from build123d import *

# Parameters (mm, degrees)
F0_W        = 50.1185376197
F0_H        = 40.0948291644
F1_DEPTH    = 50
F2_T        = -2.5
F3_T1_DEPTH = 75
F4_T1_DEPTH = 75


# Not quite as in the source:
# - a fillet or chamfer that OpenCascade refuses, or shapes differently, is made with other operations: its cross-section is extruded or revolved along the edge and cut away or added


with BuildPart() as f1:
    # F0 (on Front) → F1 (new body)
    with BuildSketch(Plane.XZ):
        with Locations((-0.201604329, 6.9467336871)):
            Rectangle(F0_W, F0_H)
    extrude(amount=F1_DEPTH)

    # F2
    f2_openings = [f1.faces().sort_by_distance(p)[0] for p in [
        (-0.201604, -25, 26.994148),
    ]]
    offset(amount=F2_T, openings=f2_openings)

    # F3: fillet of radius 5 on 1 edges, made by hand

    # F3_s2 → F3_t1 (cut)
    with BuildSketch(Plane.XZ.offset(-12.5)):
        with BuildLine():
            ThreePointArc((24.8576644808, 21.9941482693), (23.3931983867, 25.5296821752), (19.8576644808, 26.9941482693))
            Line((19.8576644808, 26.9941482693), (24.8576644808, 26.9941482693))
            Line((24.8576644808, 26.9941482693), (24.8576644808, 21.9941482693))
        make_face()
    extrude(amount=F3_T1_DEPTH, mode=Mode.SUBTRACT)

    # F4: fillet of radius 5 on 1 edges, made by hand

    # F4_s2 → F4_t1 (cut)
    with BuildSketch(Plane.XZ.offset(-12.5)):
        with BuildLine():
            ThreePointArc((-25.2608731389, 21.9941482693), (-23.7964070448, 25.5296821752), (-20.2608731389, 26.9941482693))
            Line((-20.2608731389, 26.9941482693), (-25.2608731389, 26.9941482693))
            Line((-25.2608731389, 26.9941482693), (-25.2608731389, 21.9941482693))
        make_face()
    extrude(amount=F4_T1_DEPTH, mode=Mode.SUBTRACT)


solid = f1.part
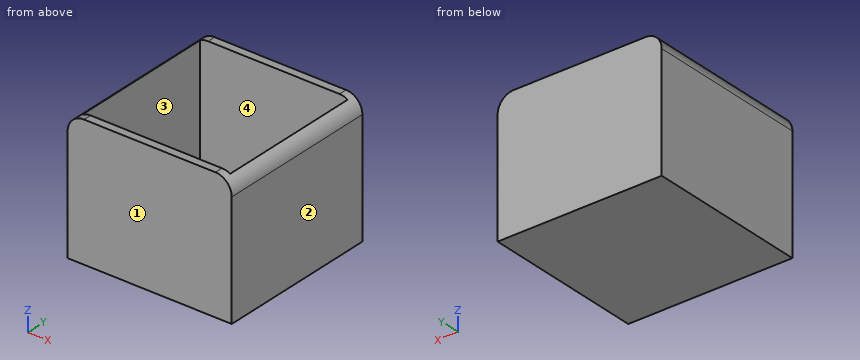
Input: part model. Units: mm. Frame: model coordinates. Face numbers are marked on the shaded views. Coordinates: 2 decimals unless noted, no trailing zeros. Write each loop counter-clockwise with the first axis right and the second up, starting at its lowest first coordinate (ties: lowest second). Pieces come first, ordered by that corner, then holes. Notation, with made-up numbers: M 65,-29.75 L 91,-29.75 A22 ccw 91,-1.75 Z; hole C 54,5 d7. An arc over 180 degrees is marked long. Answer as a JSON object with one key per item and string values. Group by question number.
(1) Contact query for a flat-ended pin moving along its axis: P1, Ø22.5, axis at x = 5.5, y = -31, coming from the +Z side. Output: stop coordinate, or through.
(2) Section B-B on x = -9.5. Output: boundary loops of the cut face in (y, z).
(3) Mould query, pull axis X, two halves, no side actions, for the marked faces 1, 2, 3 and 4. Classes: pulls with the +X half, pulls with the -X half, needs draft (parallel to the pull), parting line crosses it, or undercut.
(4) Section C-C on y = -44. Output: boundary loops of the cut face in (x, z), plus the area to 3 significant figures.
(5) Ray query, line 1 along Y through (x, z) = (5, 4.5); line 2 along X through (y, z) = (-6.5, -5); line 3 along Z through (x, y) = (18.5, -12). Return the intervals inside material, ascending. Write a range as [from, to].
(6) Section A-A on z = -5.5. Output: boundary loops of the cut face in (x, y).
Result set:
{
 "1": {"P1": "stops at z = -10.6"},
 "2": {"outline": "M -50,-13.1 L 0,-13.1 L 0,26.99 L -2.5,26.99 L -2.5,-10.6 L -47.5,-10.6 L -47.5,26.99 L -50,26.99 Z"},
 "3": {"face 1": "needs draft", "face 2": "pulls with the +X half", "face 3": "undercut", "face 4": "undercut"},
 "4": {"outline": "M -25.26,-13.1 L 24.86,-13.1 L 24.86,21.99 A5 ccw 22.36,26.32 L 22.36,-10.6 L -22.76,-10.6 L -22.76,26.32 A5 ccw -25.26,21.99 Z", "area": "304 mm2"},
 "5": {"line 1": "y = [-50, -47.5], [-2.5, 0]", "line 2": "x = [-25.26, -22.76], [22.36, 24.86]", "line 3": "z = [-13.1, -10.6]"},
 "6": {"outline": "M -25.26,-50 L 24.86,-50 L 24.86,0 L -25.26,0 Z; hole M -22.76,-47.5 L 22.36,-47.5 L 22.36,-2.5 L -22.76,-2.5 Z"}
}
